```python
from build123d import *

# Parameters (mm, degrees)
F1_DEPTH             = 12.5
F2_SIZE              = 5
F3_R                 = 2
F4_R                 = 5
F6_R                 = 5
F8_D                 = 3.7973
F8_DEPTH             = 12.62
F8_CSINK_D           = 7.7978
F8_CSINK_ANGLE       = 82
F8_TIP               = 1.1408240143
F8_ON_F7_D           = 3.7973
F8_ON_F7_DEPTH       = 12.62
F8_ON_F7_CSINK_D     = 7.7978
F8_ON_F7_CSINK_ANGLE = 82
F8_ON_F7_TIP         = 1.1408240143


with BuildPart() as f1:
    # F0 (on Top) → F1 (new body, symmetric)
    with BuildSketch(Plane.XY):
        with BuildLine():
            Line((0, 0), (35.5, 0))
            Line((35.5, 0), (35.5, -70))
            Line((35.5, -70), (38.5, -70))
            Line((38.5, -70), (38.5, 1))
            Line((38.5, 1), (-5, 1))
            Line((-5, 1), (-5, -149))
            ThreePointArc((-5, -149), (-35.1077410922, -173.4726578233), (-52.9128784748, -139))
            ThreePointArc((-52.9128784748, -139), (-51.4721155147, -129.4487973384), (-57.4954541697, -137))
            ThreePointArc((-57.4954541697, -137), (-36.1292893107, -178.3671893879), (0, -149))
            Line((0, -149), (0, 0))
        make_face()
    extrude(amount=F1_DEPTH, both=True)

    # F2
    f2_edges = [f1.edges().sort_by_distance(p)[0] for p in [
        (37, -70, 12.5),
        (37, -70, -12.5),
    ]]
    chamfer(f2_edges, length=F2_SIZE)

    # F3
    f3_edges = [f1.edges().sort_by_distance(p)[0] for p in [
        (-5, 1, 0),
        (38.5, 1, 0),
    ]]
    fillet(f3_edges, radius=F3_R)

    # F4
    f4_edges = [f1.edges().sort_by_distance(p)[0] for p in [
        (37, -65, 12.5),
        (37, -70, 7.5),
        (37, -65, -12.5),
        (37, -70, -7.5),
    ]]
    fillet(f4_edges, radius=F4_R)

    # F6
    f6_edges = [f1.edges().sort_by_distance(p)[0] for p in [
        (-57.495454, -137, 0),
        (-52.912878, -139, 0),
    ]]
    fillet(f6_edges, radius=F6_R)

    # F8
    with Locations(Plane(origin=(-5, 0, 0), x_dir=(0, -1, 0), z_dir=(-1, 0, 0))):
        with Locations((120, 0)):
            CounterSinkHole(F8_D / 2, F8_CSINK_D / 2, depth=F8_DEPTH, counter_sink_angle=F8_CSINK_ANGLE)
            with Locations((0, 0, -(F8_DEPTH + F8_TIP / 2))):  # 118° drill point
                Cone(0, F8_D / 2, F8_TIP, mode=Mode.SUBTRACT)

    # F8 on F7
    with Locations(Plane.YZ.offset(38.5)):
        with Locations((-60, 0)):
            CounterSinkHole(F8_ON_F7_D / 2, F8_ON_F7_CSINK_D / 2, depth=F8_ON_F7_DEPTH, counter_sink_angle=F8_ON_F7_CSINK_ANGLE)
            with Locations((0, 0, -(F8_ON_F7_DEPTH + F8_ON_F7_TIP / 2))):  # 118° drill point
                Cone(0, F8_ON_F7_D / 2, F8_ON_F7_TIP, mode=Mode.SUBTRACT)


solid = f1.part
```
Model file for the job. Use its own axes, mm. A direction names the side the tool comes from. Coordinates: 2 decimals unless noted, no trailing zeros. Loops run counter-clockwise (first coordinate to the right, second up) from the corner with the lowest first, then second, coordinate; pieces in that order, holes last. Notation, with made-up numbers: (33, 59) - (56, 59) arc R5 cw to (56, 67) - close; hole circle Ø5 at (64, 89.25). An arc over 180 degrees is marked (long way). Write item = value, one per line. Start each with the question number.
Item 1: Saw through at C-C, the plane x = -30. List the corners of the cut face in (y, z).
Item 2: Drop flat-ended pins along their axis: pin 1 Ø3.5 at (x, z) = (37.5, 0.5) entering from -Y; pin 2 Ø7.5 at (y, z) = (-33, 4.5) entering from -X; pin 3 Ø1.5 at (x, z) = (-16.5, 8) entering from +Y. Give the stop position or say it passes through.
Item 3: Wall check: probe 1 along Z at (x, y) = (-0.95, -120); probe 2 along X at (y, z) = (-149, 7); probe 3 along X at (y, z) = (-52, -11.5). Give the ranges that are in metal, low to high. Write a range as [from, to].
Item 4: Saw through at B-B, the plane y = -120. List the corners of the cut face in (x, z), then the cut area to 3 significant figures.
Item 5: Saw through at D-D, the plane y = -74.5. List the corners of the cut face in (x, z), then the cut area to 3 significant figures.
Item 6: Saw through at A-A, the plane y = -50.5. List the corners of the cut face in (x, z).
Item 7: Pull direction Z, two halves, no side cores. Call faces 1 (the face through (0, -76, 0)), 2 (the face through (-4, -95, 12.5)), 3 (the face through (35.845, -58.103, 0.083)): +Z half, -Z half, draft (parallel to the pull), parting line (faces both ways), or undercut.
Item 8: 3-axis set-ups, long thin cutter, end or side, ignore diameter. For faces 4 (the face through (18, 0, 0)), 5 (the face through (-51.394, -129.484, 0.175)): which of +Z, -Z, +X, -X, +Y, -Y reach the whole face in a straight line?
Answers:
q1.outline = (-179, -12.5) - (-174, -12.5) - (-174, 12.5) - (-179, 12.5) - close
q2.pin_1 = -70
q2.pin_2 = -5
q2.pin_3 = -169.54
q3.probe_1 = [-12.5, -1.9], [1.9, 12.5]
q3.probe_2 = [-60, -55], [-5, 0]
q3.probe_3 = [-5, 0], [35.5, 38.5]
q4.outline = (-5, -12.5) - (0, -12.5) - (0, -1.9) - (-2.7, -1.9) - (-5, -3.9) - close; (-5, 3.9) - (-2.7, 1.9) - (0, 1.9) - (0, 12.5) - (-5, 12.5) - close
q4.area = 101 mm2
q5.outline = (-5, -12.5) - (0, -12.5) - (0, 12.5) - (-5, 12.5) - close
q5.area = 125 mm2
q6.outline = (-5, -12.5) - (0, -12.5) - (0, 12.5) - (-5, 12.5) - close; (35.5, -12.5) - (38.5, -12.5) - (38.5, 12.5) - (35.5, 12.5) - close
q7.face_1 = draft
q7.face_2 = +Z half
q7.face_3 = undercut
q8.face_4 = +Z, -Z, -Y
q8.face_5 = +Z, -Z
